Could you check a few things on this model? Use its own coordinates, in mm. Face numbers are marked on the shaded views. A direction names the side the tool comes from. Round coordinates to 2 decimals unless told otherwise and drop trailing zeros. Order: outer loops, then holes, each group sorted by start corner. A loop starts at its lowest first (then second) coordinate and runs counter-clockwise, first axis right, second up. Notation, with made-up numbers: (-25.5, 31.25) -> (17.5, 31.25) arc R17 cw to (17.5, 38.25) -> close; hole circle Ø11 at (9, 14.25). An arc over 180 degrees is marked (long way). Put each result on its own line as item: value. Start each with the question number.
from build123d import *


with BuildPart() as part:
    # Esquisse1 → R_volution1 (revolve)
    with BuildSketch(Plane.XY, mode=Mode.PRIVATE) as r_volution1_sk:
        with BuildLine():
            Line((-6.5, 4.4), (-6.5, 4.3))
            Line((-6.5, 4.3), (-11.8, 4.3))
            Line((-11.8, 4.3), (-12.5, 3.6))
            Line((-12.5, 3.6), (-12.5, 0))
            Line((-12.5, 0), (12.5, 0))
            Line((12.5, 0), (12.5, 3.7))
            Line((12.5, 3.7), (11.8, 4.4))
            Line((11.8, 4.4), (9.5, 4.4))
            Line((9.5, 4.4), (9.5, 3.55))
            ThreePointArc((9.5, 3.55), (9.265685425, 2.984314575), (8.7, 2.75))
            Line((8.7, 2.75), (7.368165998, 2.75))
            ThreePointArc((7.368165998, 2.75), (6.954414959, 2.660390069), (6.614816325, 2.407620157))
            Line((6.614816325, 2.407620157), (6.383280582, 2.142379843))
            ThreePointArc((6.383280582, 2.142379843), (6.043681947, 1.889609931), (5.629930909, 1.8))
            Line((5.629930909, 1.8), (-0.5, 1.8))
            ThreePointArc((-0.5, 1.8), (-1.207106781, 2.092893219), (-1.5, 2.8))
            Line((-1.5, 2.8), (-1.5, 4.4))
            Line((-1.5, 4.4), (-6.5, 4.4))
        make_face()
    revolve(r_volution1_sk.sketch.rotate(Axis((-13.47216, 0, 0), (1, 0, 0)), 90), axis=Axis((-13.47216, 0, 0), (1, 0, 0)))


solid = part.part
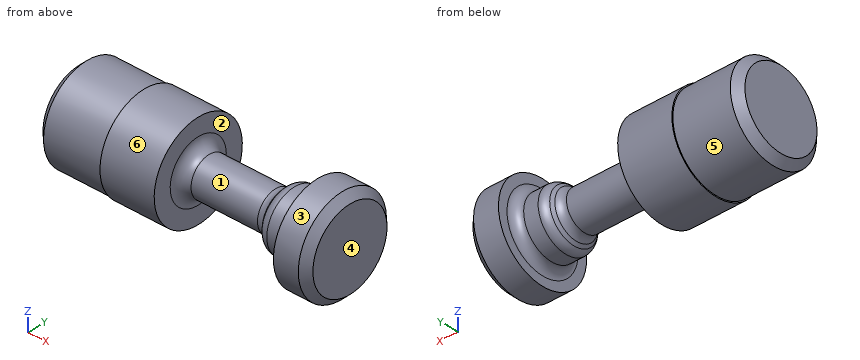
1. If we section it at D-D, the plane x = 3: Please give me the cut outline in (y, z), then the cut area to 3 significant figures.
2. I need wall thicknesses on L1, parallel to X at y = -0.5, z = -3.5; L2, parallel to X at y = -1.5, z = -2; L3, parallel to Z at x = -8.5, y = 0.25. Which ranges of each line are inside material? Lowest first, please.
3. If we section it at C-C, the plane x = -8.75: Please give me the cut outline in (y, z), then the cut area to 3 significant figures.
4. Which directions (+Z, -Z, +X, -X, +Y, -Y) give clear straight access to the entire face, cutting with the end or side of a thin tool? Please do the marked faces 5 and 6.
5. For pin 1 Ø4 at (x, z) = (-5, 0.5) entering from -Y; pin 2 Ø4 at (x, z) = (5.5, 1.5) entering from -Y; pin 3 Ø2 at (x, y) = (-5, 2.5) entering from +Z; pin 4 Ø3 at (x, z) = (5, -3) entering from -Y (3 decimals), each with a flat end and sliding along its axis, tell me the tip position at first contact or that it passes through.
6. Thinking about a two-plate mould opening in X: for the marked faces 1, 2, 3 and 4, which applies, +X half, -X half, draft (parallel to the pull), parting line (faces both ways), or undercut?
Results below:
1. outline: circle Ø3.6 at (0, 0)
1. area: 10.2 mm2
2. L1: -12.5 to -1.5, 9.5 to 12.5
2. L2: -12.5 to -1.45, 6.71 to 12.5
2. L3: -4.29 to 4.29
3. outline: circle Ø8.6 at (0, 0)
3. area: 58.1 mm2
4. face 5: -X
4. face 6: +X, -X
5. pin 1: y = -4.4
5. pin 2: y = -2.7
5. pin 3: z = 4.14
5. pin 4: y = -0.995
6. face 1: undercut
6. face 2: undercut
6. face 3: draft
6. face 4: +X half
